Verification items for the finished model (mm, model axes). Give positions to 0.01 mm unless a question says otherwise; leave off trailing zeros. Write each loop counter-clockwise with the first axis right and the second up, starting at its lowest first coordinate (ties: lowest second). Pieces come first, ordered by that corner, then holes. Notation, with made-up numbers: (23, 42) -> (48, 42) arc R23 ccw to (48, 71) -> close; hole circle Ø9 at (-34, 35). An arc over 180 degrees is marked (long way). Use CSV: the item, a comma, the result in double quotes. Start each with the question number.
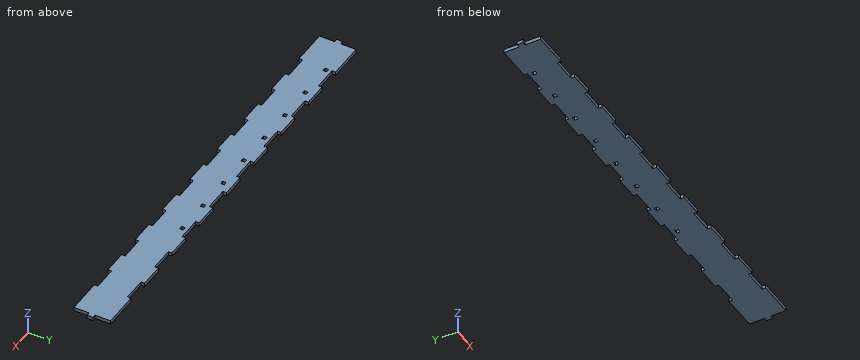
```python
from build123d import *

# Parameters (mm, degrees)
SKETCH1_W           = 3
SKETCH1_H           = 3
BOSS_EXTRUDE2_DEPTH = 3


with BuildPart() as part:
    # Sketch1 → Boss-Extrude2 (new body)
    with BuildSketch(Plane.XY):
        Polygon((28.442880719, -76.852652167), (28.442880719, -79.852652167), (8.442880719, -79.852652167), (8.442880719, -76.852652167), (-11.557119281, -76.852652167), (-11.557119281, -79.852652167), (-31.557119281, -79.852652167), (-31.557119281, -76.852652167), (-61.557119281, -76.852652167), (-61.557119281, -79.852652167), (-61.557119281, -89.852652167), (-64.557119281, -89.852652167), (-64.557119281, -94.852652167), (-61.557119281, -94.852652167), (-61.557119281, -104.852652167), (-61.557119281, -107.852652167), (-31.557119281, -107.852652167), (-31.557119281, -104.852652167), (-11.557119281, -104.852652167), (-11.557119281, -107.852652167), (8.442880719, -107.852652167), (8.442880719, -104.852652167), (28.442880719, -104.852652167), (28.442880719, -107.852652167), (48.442880719, -107.852652167), (48.442880719, -104.852652167), (68.442880719, -104.852652167), (68.442880719, -107.852652167), (88.442880719, -107.852652167), (88.442880719, -104.852652167), (108.442880719, -104.852652167), (108.442880719, -107.852652167), (128.442880719, -107.852652167), (128.442880719, -104.852652167), (148.442880719, -104.852652167), (148.442880719, -107.852652167), (168.442880719, -107.852652167), (168.442880719, -104.852652167), (188.442880719, -104.852652167), (188.442880719, -107.852652167), (208.442880719, -107.852652167), (208.442880719, -104.852652167), (228.442880719, -104.852652167), (228.442880719, -107.852652167), (248.442880719, -107.852652167), (248.442880719, -104.852652167), (268.442880719, -104.852652167), (268.442880719, -107.852652167), (298.442880719, -107.852652167), (298.442880719, -104.852652167), (298.442880719, -94.852652167), (301.442880719, -94.852652167), (301.442880719, -89.852652167), (298.442880719, -89.852652167), (298.442880719, -79.852652167), (298.442880719, -76.852652167), (268.442880719, -76.852652167), (268.442880719, -79.852652167), (248.442880719, -79.852652167), (248.442880719, -76.852652167), (228.442880719, -76.852652167), (228.442880719, -79.852652167), (208.442880719, -79.852652167), (208.442880719, -76.852652167), (188.442880719, -76.852652167), (188.442880719, -79.852652167), (168.442880719, -79.852652167), (168.442880719, -76.852652167), (148.442880719, -76.852652167), (148.442880719, -79.852652167), (128.442880719, -79.852652167), (128.442880719, -76.852652167), (108.442880719, -76.852652167), (108.442880719, -79.852652167), (88.442880719, -79.852652167), (88.442880719, -76.852652167), (68.442880719, -76.852652167), (68.442880719, -79.852652167), (48.442880719, -79.852652167), (48.442880719, -76.852652167), align=None)
        with Locations((-0.057119281, -84.352652167)):
            Rectangle(SKETCH1_W, SKETCH1_H, mode=Mode.SUBTRACT)
        with Locations((-30.057119281, -84.352652167)):
            Rectangle(SKETCH1_W, SKETCH1_H, mode=Mode.SUBTRACT)
        with Locations((29.942880719, -84.352652167)):
            Rectangle(SKETCH1_W, SKETCH1_H, mode=Mode.SUBTRACT)
        with Locations((59.942880719, -84.352652167)):
            Rectangle(SKETCH1_W, SKETCH1_H, mode=Mode.SUBTRACT)
        with Locations((89.942880719, -84.352652167)):
            Rectangle(SKETCH1_W, SKETCH1_H, mode=Mode.SUBTRACT)
        with Locations((119.942880719, -84.352652167)):
            Rectangle(SKETCH1_W, SKETCH1_H, mode=Mode.SUBTRACT)
        with Locations((149.942880719, -84.352652167)):
            Rectangle(SKETCH1_W, SKETCH1_H, mode=Mode.SUBTRACT)
        with Locations((179.942880719, -84.352652167)):
            Rectangle(SKETCH1_W, SKETCH1_H, mode=Mode.SUBTRACT)
    extrude(amount=BOSS_EXTRUDE2_DEPTH)


solid = part.part
```
(1) Thickness scan on line 1 (Y direction, x = 26, z = 1.45); line 2 (X direction, y = -98, z = 2.1); line 3 (Y direction, x = 58.5, z = 2.45). Record the ranges inside material, lowest first. Write a range as from..to.
(2) Section check A-A on z = 2.25. Give the number of separate pieces and of enclosed holes in the cut face, then the cut area to 3 significant figures.
(3) Go/stop test with flat-tipped pins: pin 1 (0.9 mm diameter, centred on y = -83.5, z = 1, fed in from +X); pin 2 (1.5 mm diameter, centred on x = 98.5, z = 2, fed in from -Y); pin 3 (0.9 mm diameter, centred on y = -84, z = 1.5, fed in from -X). Record where each tip stops, or that it passes through.
(4) Section check B-B on x = 258. Record the cut outline in (y, z), then the cut area to 3 significant figures.
(5) Section check C-C on y = -100.5. Record the cut outline in (x, z).
Data:
1,line 1,"y = -104.85..-79.85"
1,line 2,"x = -61.56..298.44"
1,line 3,"y = -104.85..-85.85, -82.85..-79.85"
2,separate pieces,"1"
2,enclosed holes,"8"
2,area,"10,200 mm2"
3,pin 1,"stops at x = 298.44"
3,pin 2,"stops at y = -104.85"
3,pin 3,"stops at x = -61.56"
4,outline,"(-104.85, 0) -> (-79.85, 0) -> (-79.85, 3) -> (-104.85, 3) -> close"
4,area,"75.0 mm2"
5,outline,"(-61.56, 0) -> (298.44, 0) -> (298.44, 3) -> (-61.56, 3) -> close"
